For this review, take the finished solid that the model builds, in its own axes (mm). A direction names the side the tool comes from. Round coordinates to 2 decimals unless told otherwise and drop trailing zeros. Order: outer loops, then holes, each group sorted by start corner. A loop starts at its lowest first (then second) coordinate and runs counter-clockwise, first axis right, second up. Notation, with made-up numbers: M 21.5,-29 L 27.5,-29 A24 cw 27.5,3 Z; hole C 64.25,13.5 d4. An arc over 180 degrees is marked long. Answer in a Markdown table with one row per item. Add a question column.
```python
from build123d import *

# Parameters (mm, degrees)
F0_W           = 18
F0_H           = 30
F1_DEPTH       = 30
F4_D           = 7
F4_DEPTH       = 15.001
F5_D           = 3.7
F5_CSINK_D     = 7
F5_CSINK_ANGLE = 90
F8_D           = 7
F8_DEPTH       = 1.001
F9_D           = 3.7
F9_CSINK_D     = 7
F9_CSINK_ANGLE = 90
F10_SIZE       = 0.99999


# Not quite as in the source:
# - a fillet or chamfer is up to 0.001 mm smaller than in the source, because OpenCascade refuses the exact size


with BuildPart() as f1:
    # F0 (on Front) → F1 (new body)
    with BuildSketch(Plane.XZ):
        with Locations((0, 15)):
            Rectangle(F0_W, F0_H)
    extrude(amount=F1_DEPTH)

    # F4 (through all, one way)
    with BuildSketch(Plane(origin=(0, -15, 0), x_dir=(1, 0, 0), z_dir=(0, 1, 0))):
        with Locations((0, -24), (0, -12)):
            Circle(F4_D / 2)
    extrude(amount=-F4_DEPTH, mode=Mode.SUBTRACT)

    # F5 (through all)
    with Locations(Plane.XZ.offset(15)):
        with Locations((0, 24), (0, 12)):
            CounterSinkHole(F5_D / 2, F5_CSINK_D / 2, counter_sink_angle=F5_CSINK_ANGLE)

    # F8 (through all, one way)
    with BuildSketch(Plane(origin=(8, 0, 0), x_dir=(0, 1, 0), z_dir=(-1, 0, 0))):
        with Locations((-25.5, -18), (-25.5, -6)):
            Circle(F8_D / 2)
    extrude(amount=-F8_DEPTH, mode=Mode.SUBTRACT)

    # F9 (through all)
    with Locations(Plane.YZ.offset(8)):
        with Locations((-25.5, 18), (-25.5, 6)):
            CounterSinkHole(F9_D / 2, F9_CSINK_D / 2, counter_sink_angle=F9_CSINK_ANGLE)

    # F10 (size 1 in the source; OpenCascade refuses exactly that, so slightly less here)
    f10_edges = [f1.edges().sort_by_distance(p)[0] for p in [
        (9, -30, 15),
        (9, -15, 30),
        (0, -30, 30),
        (9, -15, 0),
        (0, -30, 0),
    ]]
    chamfer(f10_edges, length=F10_SIZE)


solid = f1.part
```
1. For faces 5 (the cylindrical face through (8.493, -22.267, 7.341)), 6 (the cylindrical face through (-0.46, -22.4, 20.53)), 7 (the flat face through (-9, -15, 15)), list the 3-axis set-ups (+Z, -Z, +X, -X, +Y, -Y) from which the entire face can be reached by the end or side of a thin tool; tool diameter is ignored.
2. The part is to be moulded in two halves that separate along Z. For faces 1 (the cylindrical face through (0.401, -6.582, 10.194)), 2 (the flat face through (8.5, -14.3, 29.5)), 3 (the cylindrical face through (-0.759, -22.395, 15.417)), 4 (the flat face through (8.5, -14.3, 0.5)), say which applies: pulls with the +Z half, pulls with the -Z half, needs draft (parallel to the pull), parting line crosses it, or undercut.
3. To check wall thickness, follow probe 1 along Z at (x, y) = (-4, -25.5); probe 2 along Z at (x, y) = (0, -6); probe 3 along Y at (x, z) = (-2, 18). State the ranges of each line that lie inside material, in increasing order. Write a range as [from, to].
4. Consider section B-B on y = -25.5. Write out the cut boundary in (x, z), plus the area to 3 significant figures.
5. Consider section D-D on y = -14.5. Write out the cut boundary in (x, z).
6. Clearance check with flat-ended pins moving along their axes: pin 1 Ø5 at (x, z) = (0, 24) entering from -Y; pin 2 Ø9 at (y, z) = (-25.5, 18) entering from -X; pin 3 Ø5.5 at (x, z) = (0, 12) entering from -Y; pin 4 Ø6 at (y, z) = (-25.5, 18) entering from +X. State where each tip first meets the part, or that it passes through.
7. Consider section A-A on x = 0. Write out the cut boundary in (y, z), plus the area to 3 significant figures.
Solved:
| question | item | result |
|---|---|---|
| 1 | face 5 | +X |
| 1 | face 6 | -Y |
| 1 | face 7 | +Z, -Z, -X, +Y, -Y |
| 2 | face 1 | undercut |
| 2 | face 2 | pulls with the +Z half |
| 2 | face 3 | undercut |
| 2 | face 4 | pulls with the -Z half |
| 3 | probe 1 | z = [0, 4.15], [7.85, 16.15], [19.85, 30] |
| 3 | probe 2 | z = [0, 10.15], [13.85, 22.15], [25.85, 30] |
| 3 | probe 3 | y = [-30, -27.35], [-23.65, 0] |
| 4 | outline | M -9,0 L 8,0 L 9,1 L 9,2.5 L 8,2.5 L 6.35,4.15 L -9,4.15 Z; M -9,7.85 L 6.35,7.85 L 8,9.5 L 9,9.5 L 9,14.5 L 8,14.5 L 6.35,16.15 L -9,16.15 Z; M -9,19.85 L 6.35,19.85 L 8,21.5 L 9,21.5 L 9,29 L 8,30 L -9,30 Z; hole C 0,12 d7; hole C 0,24 d7 |
| 4 | area | 317 mm^2 |
| 5 | outline | M -9,0 L 8,0 L 9,1 L 9,29 L 8,30 L -9,30 Z; hole C 0,12 d6; hole C 0,24 d6 |
| 6 | pin 1 | stops at y = -14 |
| 6 | pin 2 | stops at x = -9 |
| 6 | pin 3 | stops at y = -14.25 |
| 6 | pin 4 | stops at x = 7.5 |
| 7 | outline | M -30,1 L -29,0 L 0,0 L 0,10.15 L -13.35,10.15 L -15,8.5 L -30,8.5 Z; M -30,15.5 L -15,15.5 L -13.35,13.85 L 0,13.85 L 0,22.15 L -13.35,22.15 L -15,20.5 L -30,20.5 Z; M -30,27.5 L -15,27.5 L -13.35,25.85 L 0,25.85 L 0,30 L -29,30 L -30,29 Z; hole C -25.5,6 d3.7; hole C -25.5,18 d3.7 |
| 7 | area | 551 mm^2 |
